The listing builds one solid part. Answer for the finished solid, in the listing's coordinates (mm). Face numbers are marked on the shaded views. Round coordinates to 2 decimals unless told otherwise and drop trailing zeros. Loops run counter-clockwise (first coordinate to the right, second up) from the corner with the lowest first, then second, coordinate; pieces in that order, holes last. Notation, with made-up numbers: (-13.5, 5.25) - (38.5, 5.25) arc R12 cw to (38.5, 14.25) - close; hole circle Ø8 at (52, 59). An arc over 180 degrees is marked (long way). Write item = value, one per line. Start each with the question number.
1) Section C-C, the plane z = -64 is taken. Determine the outline of the cut face in (x, y), and give its area (3 significant figures).
2) Straight lines are drawn through the part: line 1 along Z through (x, y) = (-4, 0); line 2 along X through (y, z) = (0, -69.1). For each, find the intervals that lie inside material, in ascending order.
3) For a pull along Z with two mould halves and no side action, classify the marked faces 1, 2 and 3 as released by +Z, released by -Z, zero draft, split by the parting line, or undercut.
4) Given pin 1 Ø8 at (x, z) = (-8, -30.5) entering from +Y; pin 2 Ø6 at (y, z) = (-6.5, -60.5) entering from +X; pin 3 Ø3 at (x, z) = (-6.5, -44.5) entering from +Y; pin 4 Ø8 at (y, z) = (2, -28.5) entering from +X, each flat-ended and moving along its own axis, determine where each tip first touches the part or whether it passes through.
from build123d import *


with BuildPart() as part:
    # Sketch1 → Revolve1 (revolve)
    with BuildSketch(Plane(origin=(0, 0, 0), x_dir=(1, 0, 0), z_dir=(0, 1, 0))):
        with BuildLine():
            Line((0, 70.09), (4.39217757, 70.09))
            ThreePointArc((4.39217757, 70.09), (4.487086316, 70.066046386), (4.559260987, 69.9999233))
            Line((4.559260987, 69.9999233), (5.440739013, 68.6600767))
            ThreePointArc((5.440739013, 68.6600767), (5.512913684, 68.593953614), (5.60782243, 68.57))
            Line((5.60782243, 68.57), (6.955, 68.57))
            Line((6.955, 68.57), (6.955, 68.67))
            Line((6.955, 68.67), (7.745, 68.67))
            Line((7.745, 68.67), (7.745, 68.97))
            Line((7.745, 68.97), (8.1, 68.97))
            Line((8.1, 68.97), (8.1, 69.15596492))
            ThreePointArc((8.1, 69.15596492), (8.127103293, 69.256497147), (8.201067285, 69.32978183))
            ThreePointArc((8.201067285, 69.32978183), (9.040599123, 69.672998391), (9.94, 69.79))
            ThreePointArc((9.94, 69.79), (10.350121933, 69.620121933), (10.52, 69.21))
            Line((10.52, 69.21), (10.52, 0.4))
            ThreePointArc((10.52, 0.4), (10.402842712, 0.117157288), (10.12, 0))
            Line((10.12, 0), (0, 0))
            Line((0, 0), (0, 68.27))
            Line((0, 68.27), (5.338266355, 68.27))
            Line((5.338266355, 68.27), (4.338266355, 69.79))
            Line((4.338266355, 69.79), (0, 69.79))
            Line((0, 69.79), (0, 70.09))
        make_face()
    revolve(axis=Axis((0, 0, 0), (0, 0, -1)))


solid = part.part
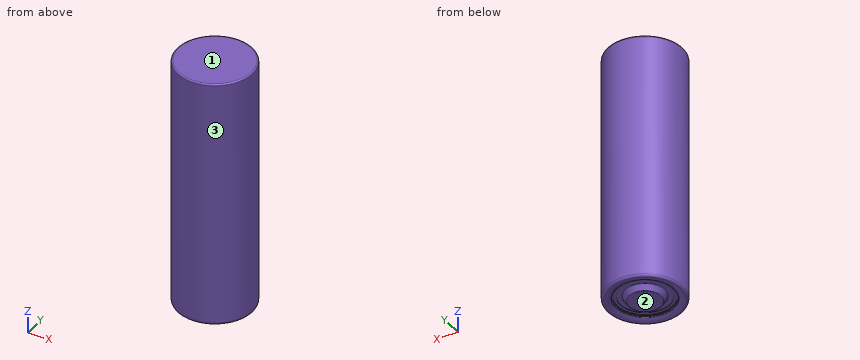
Geometry check:
q1.outline = circle Ø21.04 at (0, 0)
q1.area = 348 mm2
q2.line_1 = -70.09 to -69.79, -68.27 to 0
q2.line_2 = -10.52 to -8.1, -5.15 to -4.79, 4.79 to 5.15, 8.1 to 10.52
q3.face_1 = released by +Z
q3.face_2 = released by -Z
q3.face_3 = zero draft
q4.pin_1 = 9.73
q4.pin_2 = 9.92
q4.pin_3 = 9.26
q4.pin_4 = 10.52
